from build123d import *

# Parameters (mm, degrees)
SKETCH1_W                 = 401
SKETCH1_H                 = 111
BOSS_EXTRUDE1_DEPTH       = 10.5
CUT_EXTRUDE1_DEPTH        = 3
CUT_EXTRUDE2_DEPTH        = 417.550165046
BOSS_EXTRUDE2_DEPTH       = 7.5
FILLET4_R                 = 2
SKETCH21_W                = 4
SKETCH21_H                = 96
BOSS_EXTRUDE3_DEPTH       = 7.5
FILLET5_R                 = 2
FILLET6_R                 = 4
CHAMFER2_SIZE             = 0.5
FILLET7_R                 = 3.175
M2X0_4_TAPPED_HOLE2_D     = 1.6
M2X0_4_TAPPED_HOLE2_DEPTH = 5.75
M2X0_4_TAPPED_HOLE2_TIP   = 0.480688495
M2X0_4_TAPPED_HOLE3_D     = 1.6
M2X0_4_TAPPED_HOLE3_DEPTH = 5.75
M2X0_4_TAPPED_HOLE3_TIP   = 0.480688495
CUT_EXTRUDE3_DEPTH        = 3


with BuildPart() as part:
    # Sketch1 → Boss-Extrude1 (new body)
    with BuildSketch(Plane(origin=(0, 0, 0), x_dir=(1, 0, 0), z_dir=(0, 1, 0))):
        with Locations((200.5, 55.5)):
            Rectangle(SKETCH1_W, SKETCH1_H)
    extrude(amount=BOSS_EXTRUDE1_DEPTH)

    # Sketch2 → Cut-Extrude1 (cut)
    with BuildSketch(Plane.XZ):
        with BuildLine():
            Line((8, -2), (393, -2))
            ThreePointArc((393, -2), (397.242640687, -3.757359313), (399, -8))
            Line((399, -8), (399, -103))
            ThreePointArc((399, -103), (397.242640687, -107.242640687), (393, -109))
            Line((393, -109), (8, -109))
            ThreePointArc((8, -109), (3.757359313, -107.242640687), (2, -103))
            Line((2, -103), (2, -8))
            ThreePointArc((2, -8), (3.757359313, -3.757359313), (8, -2))
        make_face()
    extrude(amount=-CUT_EXTRUDE1_DEPTH, mode=Mode.SUBTRACT)

    # Sketch3 → Cut-Extrude2 (cut, through all)
    with BuildSketch(Plane.XZ.offset(9.3)):
        with BuildLine():
            Line((9.5, -7.5), (391.5, -7.5))
            ThreePointArc((391.5, -7.5), (392.914213562, -8.085786438), (393.5, -9.5))
            Line((393.5, -9.5), (393.5, -101.5))
            ThreePointArc((393.5, -101.5), (392.914213562, -102.914213562), (391.5, -103.5))
            Line((391.5, -103.5), (9.5, -103.5))
            ThreePointArc((9.5, -103.5), (8.085786438, -102.914213562), (7.5, -101.5))
            Line((7.5, -101.5), (7.5, -9.5))
            ThreePointArc((7.5, -9.5), (8.085786438, -8.085786438), (9.5, -7.5))
        make_face()
    extrude(amount=-CUT_EXTRUDE2_DEPTH, mode=Mode.SUBTRACT)

    # Sketch20 → Boss-Extrude2 (add)
    with BuildSketch(Plane(origin=(0, 10.5, 0), x_dir=(1, 0, 0), z_dir=(0, 1, 0))):
        with BuildLine():
            Line((327, 7.5), (335.5, 7.5))
            Line((335.5, 7.5), (335.5, 25.5))
            ThreePointArc((335.5, 25.5), (335.207106781, 26.207106781), (334.5, 26.5))
            Line((334.5, 26.5), (328, 26.5))
            ThreePointArc((328, 26.5), (327.292893219, 26.207106781), (327, 25.5))
            Line((327, 25.5), (327, 7.5))
        make_face()
    extrude(amount=-BOSS_EXTRUDE2_DEPTH)

    # Fillet4
    fillet4_edges = [part.edges().sort_by_distance(p)[0] for p in [
        (335.5, 6.75, -7.5),
        (327, 6.75, -7.5),
    ]]
    fillet(fillet4_edges, radius=FILLET4_R)

    # Sketch21 → Boss-Extrude3 (add)
    with BuildSketch(Plane(origin=(0, 10.5, 0), x_dir=(1, 0, 0), z_dir=(0, 1, 0))):
        with Locations((86.5, 55.5)):
            Rectangle(SKETCH21_W, SKETCH21_H)
    extrude(amount=-BOSS_EXTRUDE3_DEPTH)

    # Fillet5
    fillet5_edges = [part.edges().sort_by_distance(p)[0] for p in [
        (88.5, 6.75, -7.5),
        (88.5, 6.75, -103.5),
        (84.5, 6.75, -103.5),
        (84.5, 6.75, -7.5),
    ]]
    fillet(fillet5_edges, radius=FILLET5_R)

    # Fillet6
    fillet6_edges = [part.edges().sort_by_distance(p)[0] for p in [
        (0, 5.25, -111),
        (401, 5.25, -111),
        (401, 5.25, 0),
        (0, 5.25, 0),
    ]]
    fillet(fillet6_edges, radius=FILLET6_R)

    # Chamfer2
    chamfer2_edges = [part.edges().sort_by_distance(p)[0] for p in [
        (88.5, 10.5, -55.5),
        (84.5, 10.5, -55.5),
        (46, 10.5, -7.5),
        (241, 10.5, -103.5),
        (89.085786438, 10.5, -8.085786438),
        (83.914213562, 10.5, -8.085786438),
        (83.914213562, 10.5, -102.914213562),
        (89.085786438, 10.5, -102.914213562),
        (392.914213562, 10.5, -8.085786438),
        (393.5, 10.5, -55.5),
        (392.914213562, 10.5, -102.914213562),
        (46, 10.5, -103.5),
        (8.085786438, 10.5, -102.914213562),
        (7.5, 10.5, -55.5),
        (8.085786438, 10.5, -8.085786438),
        (364.5, 10.5, -7.5),
        (327, 10.5, -17.5),
        (335.207106781, 10.5, -26.207106781),
        (331.25, 10.5, -26.5),
        (327.292893219, 10.5, -26.207106781),
        (207.75, 10.5, -7.5),
        (335.5, 10.5, -17.5),
        (326.414213562, 10.5, -8.085786438),
        (336.085786438, 10.5, -8.085786438),
    ]]
    chamfer(chamfer2_edges, length=CHAMFER2_SIZE)

    # Fillet7
    fillet7_edges = [part.edges().sort_by_distance(p)[0] for p in [
        (0, 10.5, -55.5),
        (200.5, 10.5, -111),
        (200.5, 10.5, 0),
        (401, 10.5, -55.5),
        (1.171572875, 10.5, -1.171572875),
        (399.828427125, 10.5, -1.171572875),
        (399.828427125, 10.5, -109.828427125),
        (1.171572875, 10.5, -109.828427125),
    ]]
    fillet(fillet7_edges, radius=FILLET7_R)

    # M2x0.4 Tapped Hole2
    with Locations(Plane(origin=(5.375, 3, -5.375), x_dir=(0, 0, -1), z_dir=(0, -1, 0))):
        with Locations((0, 0), (0, 130), (0, 260.25), (0, 390.25), (100.25, 390.25), (100.25, 260.25), (100.25, 130), (100.25, 0)):
            Hole(M2X0_4_TAPPED_HOLE2_D / 2, depth=M2X0_4_TAPPED_HOLE2_DEPTH)
            with Locations((0, 0, -(M2X0_4_TAPPED_HOLE2_DEPTH + M2X0_4_TAPPED_HOLE2_TIP / 2))):  # 118° drill point
                Cone(0, M2X0_4_TAPPED_HOLE2_D / 2, M2X0_4_TAPPED_HOLE2_TIP, mode=Mode.SUBTRACT)

    # M2x0.4 Tapped Hole3
    with Locations(Plane(origin=(70.375, 3, -5.375), x_dir=(0, 0, -1), z_dir=(0, -1, 0))):
        with Locations((0, 0), (0, 130.125), (0, 260.25), (50.125, 325.25), (100.25, 260.25), (100.25, 130.125), (100.25, 0), (50.125, -65)):
            Hole(M2X0_4_TAPPED_HOLE3_D / 2, depth=M2X0_4_TAPPED_HOLE3_DEPTH)
            with Locations((0, 0, -(M2X0_4_TAPPED_HOLE3_DEPTH + M2X0_4_TAPPED_HOLE3_TIP / 2))):  # 118° drill point
                Cone(0, M2X0_4_TAPPED_HOLE3_D / 2, M2X0_4_TAPPED_HOLE3_TIP, mode=Mode.SUBTRACT)

    # Sketch27 → Cut-Extrude3 (cut)
    with BuildSketch(Plane.XZ):
        with BuildLine():
            Line((393, -1.75), (8, -1.75))
            ThreePointArc((8, -1.75), (3.580582618, -3.580582618), (1.75, -8))
            Line((1.75, -8), (1.75, -103))
            ThreePointArc((1.75, -103), (3.580582618, -107.419417382), (8, -109.25))
            Line((8, -109.25), (393, -109.25))
            ThreePointArc((393, -109.25), (397.419417382, -107.419417382), (399.25, -103))
            Line((399.25, -103), (399.25, -8))
            ThreePointArc((399.25, -8), (397.419417382, -3.580582618), (393, -1.75))
        make_face()
    extrude(amount=-CUT_EXTRUDE3_DEPTH, mode=Mode.SUBTRACT)


solid = part.part
Could you check a few things on this model? Use its own coordinates, in mm. A direction names the side the tool comes from. Give positions to 0.01 mm unless a question says otherwise; leave off trailing zeros. Write each loop counter-clockwise with the first axis right and the second up, starting at its lowest first coordinate (ties: lowest second). Pieces come first, ordered by that corner, then holes. Notation, with made-up numbers: (-17.75, 63.25) -> (0.25, 63.25) arc R17 cw to (0.25, 82.25) -> close; hole circle Ø10 at (-20.75, -21). An arc over 180 degrees is marked (long way). Answer as CSV lines item,"result". Start each with the question number.
(1) Which directions (+Z, -Z, +X, -X, +Y, -Y) give clear straight access to the entire face, cutting with the end or side of a thin tool? Please do faces 1 (the face through (214, 10.5, -5)), 2 (the face through (3.53, 1.48, -107.37)), 3 (the face through (243, 6, -103.5)).
(2) I'm going to push flat-ended pins straight in: pin 1 Ø1.8 at (x, z) = (5.375, -105.625) entering from -Y; pin 2 Ø1.4 at (x, z) = (200.5, -5.375) entering from -Y. Where does each tip first touch, or does it pass through?
(3) If we section it at A-A, the plane x = 372: Write out the boundary of the cut face in (y, z) (3 decimals), and give its area (3 significant figures).
(4) If we mould it in two halves opening along X, with no side actions, what happens to faces 4 (the face through (198, 4, 0)), 5 (the face through (401, 4, -55)), 6 (the face through (47, 6, -103.5))? For each: +X half, -X half, draft (parallel to the pull), parting line (faces both ways), or undercut.
(5) If we section it at B-B, the plane z = -83.5: Write out the boundary of the cut face in (x, y) (3 decimals).
(6) If we section it at C-C, the plane z = -17.5: Write out the boundary of the cut face in (x, y) (3 decimals), and give its area (3 significant figures).
(7) Please list where these lines run through material, in increasing order: line 1 (X direction, y = 4.75, z = -99.5); line 2 (X direction, y = 5.7, z = -55.5) (3 decimals); line 3 (X direction, y = 7.25, z = -24).
Answer list:
1,face 1,"+Z, -Z, +X, -X, +Y"
1,face 2,"-Y"
1,face 3,"+Y, -Y"
2,pin 1,"y = 3"
2,pin 2,"y = 8.81"
3,outline,"(0, -111) -> (7.325, -111) arc R3.175 ccw to (10.5, -107.825) -> (10.5, -104) -> (10, -103.5) -> (3, -103.5) -> (3, -109.25) -> (0, -109.25) -> close; (0, -1.75) -> (3, -1.75) -> (3, -7.5) -> (10, -7.5) -> (10.5, -7) -> (10.5, -3.175) arc R3.175 ccw to (7.325, 0) -> (0, 0) -> close"
3,area,"118 mm^2"
4,face 4,"draft"
4,face 5,"+X half"
4,face 6,"undercut"
5,outline,"(0, 0) -> (1.75, 0) -> (1.75, 3) -> (7.5, 3) -> (7.5, 10) -> (7, 10.5) -> (3.175, 10.5) arc R3.175 ccw to (0, 7.325) -> close; (84.5, 3) -> (88.5, 3) -> (88.5, 10) -> (88, 10.5) -> (85, 10.5) -> (84.5, 10) -> close; (393.5, 3) -> (399.25, 3) -> (399.25, 0) -> (401, 0) -> (401, 7.325) arc R3.175 ccw to (397.825, 10.5) -> (394, 10.5) -> (393.5, 10) -> close"
6,outline,"(0, 0) -> (1.75, 0) -> (1.75, 3) -> (7.5, 3) -> (7.5, 10) -> (7, 10.5) -> (3.175, 10.5) arc R3.175 ccw to (0, 7.325) -> close; (84.5, 3) -> (88.5, 3) -> (88.5, 10) -> (88, 10.5) -> (85, 10.5) -> (84.5, 10) -> close; (327, 3) -> (335.5, 3) -> (335.5, 10) -> (335, 10.5) -> (327.5, 10.5) -> (327, 10) -> close; (393.5, 3) -> (399.25, 3) -> (399.25, 0) -> (401, 0) -> (401, 7.325) arc R3.175 ccw to (397.825, 10.5) -> (394, 10.5) -> (393.5, 10) -> close"
6,area,"212 mm^2"
7,line 1,"0 to 7.5, 84.5 to 88.5, 393.5 to 401"
7,line 2,"0 to 4.575, 6.175 to 7.5, 84.5 to 88.5, 393.5 to 394.825, 396.425 to 401"
7,line 3,"0 to 7.5, 84.5 to 88.5, 327 to 335.5, 393.5 to 401"
